Work out the finished part from the listing and answer in its coordinate system (mm). Coordinates: 2 decimals unless noted, no trailing zeros. Order: outer loops, then holes, each group sorted by start corner. A loop starts at its lowest first (then second) coordinate and runs counter-clockwise, first axis right, second up. Notation, with made-up numbers: M 24,23.5 L 33,23.5 A20 ccw 33,31.5 Z; hole C 13,-29.75 d7. An arc over 180 degrees is marked long. Use a Markdown table: item, result.
Autodesk Inventor part; units mm, degrees
ref_plane "YZ Plane" through (0, 0, 0) normal (1, 0, 0) x (0, 1, 0)
ref_plane "XZ Plane" through (0, 0, 0) normal (0, 1, 0) x (-1, 0, 0)
ref_plane "XY Plane" through (0, 0, 0) normal (0, 0, 1) x (1, 0, 0)
sketch "Sketch1" plane through (0, 0, 0) normal (1, 0, 0) x (0, 1, 0)
  point P0 (0, 0)
sketch "Sketch2" plane through (0, 0, 0) normal (0, 0, 1) x (1, 0, 0)
  circle A0 centre (13.979, 17.0432) radius 2.3368
  circle A1 centre (13.725, -33.7568) radius 2.3368
  circle A2 centre (-87.875, -33.7568) radius 2.3368
  circle A3 centre (-87.875, 17.0432) radius 2.3368
  line L0 (-87.621, -39.5988) -> (13.471, -39.5988)
  arc A4 (-93.971, -33.2488) -> (-87.621, -39.5988) centre (-87.621, -33.2488) ccw
  line L1 (-93.971, 17.0432) -> (-93.971, -33.2488)
  arc A5 (-87.621, 23.3932) -> (-93.971, 17.0432) centre (-87.621, 17.0432) ccw
  line L2 (13.471, 23.3932) -> (-87.621, 23.3932)
  arc A6 (19.821, 17.0432) -> (13.471, 23.3932) centre (13.471, 17.0432) ccw
  line L3 (19.821, -33.2488) -> (19.821, 17.0432)
  arc A7 (13.471, -39.5988) -> (19.821, -33.2488) centre (13.471, -33.2488) ccw
  circle A8 centre (13.725, -33.7568) radius 2.3368
  circle A9 centre (13.979, 17.0432) radius 2.3368
  circle A10 centre (-87.875, -33.7568) radius 2.3368
  circle A11 centre (-87.875, 17.0432) radius 2.3368
  point P0 (0, 0)
extrude "Extrusion1" add sketch "Sketch2" along normal blind 1.5875
sketch "Sketch3" plane through (19.821, -33.2488, 0) normal (1, 0, 0) x (0, 0, -1)
  circle A0 centre (3.7949, -1.7964) radius 3.3655
  circle A1 centre (3.7949, -1.7964) radius 4.445
  line L0 (3.1599, 2.6031) -> (-0.6501, 2.4684)
  line L1 (-0.6501, 2.4684) -> (-0.6501, -1.7964)
  line L2 (-0.6501, -1.7964) -> (-0.493, -6.2414)
  line L3 (-0.493, -6.2414) -> (3.7949, -6.2414)
  line L4 (0, 0) -> (0, 50.292)
  line L5 (7.1604, -1.7964) -> (8.2399, -1.7964)
  line L6 (6.8216, -0.3249) -> (7.744, 0.2439)
  line L7 (6.8216, -3.2678) -> (7.8694, -3.5728)
  point P0 (0, 33.2488)
  point P1 (0, 2.4914)
  point P2 (0, 1.3549)
  point P3 (-0.6391, -2.1102)
  point P4 (0, 0.5182)
  dimension "d2" = 6.731
  dimension "d3" = 8.89
extrude "Extrusion2" add sketch "Sketch3" against normal up to surface (113.792 mm away) contours L5 A1 L7 A0 | A0 L6 A1 L5 | A0 L7 A1 L6 | A1 L4 L0
sketch "Sketch4" plane through (0, 0, 1.5875) normal (0, 0, 1) x (1, 0, 0)
  circle A0 centre (13.725, -33.7568) radius 2.3368
  line L0 (19.821, -39.4902) -> (-93.971, -39.4902)
  line L1 (19.821, -39.4902) -> (19.821, -30.6002)
  line L2 (19.821, -30.7575) -> (-93.971, -30.7575)
  line L3 (19.821, -39.4902) -> (-93.971, -39.4902)
  line L4 (-93.971, -39.4902) -> (-93.971, -30.7575)
  line L5 (-93.971, -30.7575) -> (19.821, -30.7575)
  line L6 (19.821, -30.7575) -> (19.821, -39.4902)
  circle A1 centre (-87.875, -33.7568) radius 2.3368
  circle A2 centre (-87.875, 17.0432) radius 2.3368
  circle A3 centre (-87.875, 17.0432) radius 2.921
  circle A4 centre (13.979, 17.0432) radius 2.3368
  circle A5 centre (13.979, 17.0432) radius 2.921
  point P0 (0, 0)
  point P1 (19.821, -33.2488)
  point P2 (19.821, -30.6458)
  dimension "d6" = 5.842
  dimension "d7" = 5.842
extrude "Extrusion3" add sketch "Sketch4" against normal up to surface contours A0 | L0 L4 L2 L1 | A1
sketch "Sketch5" plane through (19.821, 17.0432, 1.5875) normal (1, 0, 0) x (0, 0, -1)
  line L0 (0, -56.5334) -> (0, -56.642)
  line L1 (0, -56.5334) -> (1.6302, -56.5334)
  line L2 (1.6302, -56.5334) -> (1.6302, -56.6709)
  line L3 (1.6302, -56.6709) -> (0, -56.6709)
  line L4 (0, -56.6709) -> (0, -56.5334)
  point P0 (1.5875, -17.0432)
extrude "Extrusion4" cut sketch "Sketch5" against normal blind 136.017
fillet "Fillet1" radius 1.5875 1 edges at (-37.075, -39.4902, 1.5875)
sketch "Sketch6" plane through (-93.971, 17.0432, 0) normal (-1, 0, 0) x (0, 0, 1)
  circle A0 centre (-3.7949, -52.0884) radius 3.3655
  line L0 (-7.1604, -52.0884) -> (-8.2399, -52.0884)
  arc A1 (-3.1599, -47.6889) -> (-3.7949, -56.5334) centre (-3.7949, -52.0884) ccw
  line L1 (-7.4629, -53.118) -> (-8.0595, -53.3483)
  line L2 (-7.4629, -51.0587) -> (-8.0595, -50.8284)
  point P0 (0, -17.0432)
  point P1 (-7.4631, -51.0586)
  point P2 (-8.0577, -50.8291)
  point P3 (-8.0577, -53.3476)
  point P4 (-7.4631, -53.1181)
extrude "Extrusion6" cut sketch "Sketch3" against normal blind 115.8875 contours L5 A1 L7 A0 | A0 L6 A1 L5
properties part number "plate holder holder"
1. Flat-ended cylindrical pins translate along their axes: P1, Ø4, axis at y = -35.05, z = -3.79, coming from the -X side; P2, Ø3, axis at x = -51, y = -17.5, coming from the -Z side. Find the tip coordinate at first contact, or state that the pin passes through.
Answers below:
| item | result |
|---|---|
| P1 | through |
| P2 | z = 0 |
2. For a pull along X with two mould halves and no side action, classify faces 1 (the face through (17.911, 21.582, 0.783)), 2 (the face through (13.675, 14.726, 0.783)), 3 (the face through (-90.21, 16.94, 0.78)), 4 (the face through (-36, -39.49, -2)) as +X half, -X half, draft (parallel to the pull), parting line (faces both ways), or undercut.
Answers below:
| item | result |
|---|---|
| face 1 | +X half |
| face 2 | undercut |
| face 3 | undercut |
| face 4 | draft |
3. Section B-B on z = -1.5 is taken. Determine the outline of the cut face in (x, y), then the cut area to 3 significant figures.
Answers below:
| item | result |
|---|---|
| outline | M -93.97,-39.49 L 19.82,-39.49 L 19.82,-37.51 L -93.97,-37.51 Z; M -93.97,-32.58 L 19.82,-32.58 L 19.82,-30.7 L -93.97,-30.7 Z |
| area | 440 mm² |
4. Find the intervals of material crossed by probe 1 along Y at (x, z) = (-29.5, -3.5); probe 2 along Y at (x, z) = (13, -6.25); probe 3 along Z at (x, y) = (-79.5, -16), in increasing order.
Answers below:
| item | result |
|---|---|
| probe 1 | -39.49 to -38.4, -31.69 to -30.61 |
| probe 2 | -38.75 to -37.35, -32.74 to -31.34 |
| probe 3 | 0 to 1.59 |
5. Section D-D on y = -35 is taken. Determine the outline of the cut face in (x, z), then the cut area to 3 significant figures.
Answers below:
| item | result |
|---|---|
| outline | M -93.97,-0.43 L 19.82,-0.43 L 19.82,1.59 L -93.97,1.59 Z |
| area | 230 mm² |
6. Section C-C on y = -15 is taken. Determine the outline of the cut face in (x, z).
Answers below:
| item | result |
|---|---|
| outline | M -93.97,0 L 19.82,0 L 19.82,1.59 L -93.97,1.59 Z |
7. Section A-A on x = 8 is taken. Determine the outline of the cut face in (y, z) (1 decimal).
Answers below:
| item | result |
|---|---|
| outline | M -39.5,-3.8 A4.4 ccw -36.8,-7.9 L -36.5,-6.8 A3.4 cw long -33.6,-6.8 L -33,-7.7 A4.4 ccw -30.6,-3.2 L -30.8,0 L 23.4,0 L 23.4,1.6 L -37.9,1.6 A1.6 ccw -39.5,0 Z |
